Could you check a few things on this model? Use its own coordinates, in mm. Face numbers are marked on the shaded views. Round coordinates to 2 decimals unless told otherwise and drop trailing zeros. Loops run counter-clockwise (first coordinate to the right, second up) from the corner with the lowest first, then second, coordinate; pieces in that order, holes last. Notation, with made-up numbers: (10.25, 14) -> (68.25, 14) arc R18 cw to (68.25, 45) -> close; hole circle Ø1 at (2.25, 84.5). An arc over 180 degrees is marked (long way). Put each result on its own line as item: value. Start each with the question number.
1. I'm going to push flat-ended pins straight in: P1, Ø4, axis at y = -7, z = 5, coming from the -X side; P2, Ø4, axis at y = 7, z = 76.5, coming from the +X side; P3, Ø1, axis at x = -1, z = 60.5, coming from the +Y side. Where does each tip first touch, or does it pass through?
2. Imagine slicing it at B-B, the plane x = 0. Please give me the cut outline in (y, z), and give its area (3 significant figures).
3. I need wall thicknesses on line 1 (Z direction, x = 15.5, y = 4); line 2 (Y direction, x = 13, z = 103.6); line 3 (Y direction, x = -13, z = 101.8). Which ranges of each line are inside material? Lowest first, please. Write a range as [from, to].
4. Imagine slicing it at D-D, the plane x = 12.5. Please give me the cut outline in (y, z).
5. Imagine slicing it at A-A, the plane x = -13. Please give me the cut outline in (y, z), and give its area (3 significant figures).
6. If we mould it in two halves opening along Z, with no side actions, what happens to the marked faces 1, 2, 3 and 4? For each: pulls with the +Z half, pulls with the -Z half, needs draft (parallel to the pull), parting line crosses it, or undercut.
```python
from build123d import *

# Parameters (mm, degrees)
ESQUISSE1_R             = 10
BOSS_EXTRU_1_DEPTH      = 100
ESQUISSE2_R             = 17.5
BOSS_EXTRU_2_DEPTH      = 30
ESQUISSE3_W             = 40
ESQUISSE3_H             = 40
BOSS_EXTRU_3_DEPTH      = 5
ESQUISSE4_R             = 2.5
ENL_V_MAT_EXTRU_1_DEPTH = 5
ESQUISSE5_OUTSIDE_W     = 71.274
ESQUISSE5_OUTSIDE_H     = 71.274
ESQUISSE5_OUTSIDE_R     = 10
ENL_V_MAT_EXTRU_3_DEPTH = 20


with BuildPart() as part:
    # Esquisse1 → Boss.-Extru.1 (new body)
    with BuildSketch(Plane.XY):
        Circle(ESQUISSE1_R)
    extrude(amount=BOSS_EXTRU_1_DEPTH)

    # Esquisse2 → Boss.-Extru.2 (add)
    with BuildSketch(Plane(origin=(0, 0, 0), x_dir=(-1, 0, 0), z_dir=(0, 0, -1))):
        Circle(ESQUISSE2_R)
    extrude(amount=BOSS_EXTRU_2_DEPTH)

    # Esquisse3 → Boss.-Extru.3 (add)
    with BuildSketch(Plane.XY.offset(100)):
        Rectangle(ESQUISSE3_W, ESQUISSE3_H)
    extrude(amount=BOSS_EXTRU_3_DEPTH)

    # Esquisse4 → Enlèv. mat.-Extru.1 (cut)
    with BuildSketch(Plane.XY.offset(105)):
        with Locations((-13, 13)):
            Circle(ESQUISSE4_R)
        with Locations((13, -13)):
            Circle(ESQUISSE4_R)
    extrude(amount=-ENL_V_MAT_EXTRU_1_DEPTH, mode=Mode.SUBTRACT)

    # Esquisse5 outside → Enlèv. mat.-Extru.3 (cut)
    with BuildSketch(Plane.XY):
        Rectangle(ESQUISSE5_OUTSIDE_W, ESQUISSE5_OUTSIDE_H)
        Circle(ESQUISSE5_OUTSIDE_R, mode=Mode.SUBTRACT)
    extrude(amount=-ENL_V_MAT_EXTRU_3_DEPTH, mode=Mode.SUBTRACT)


solid = part.part
```
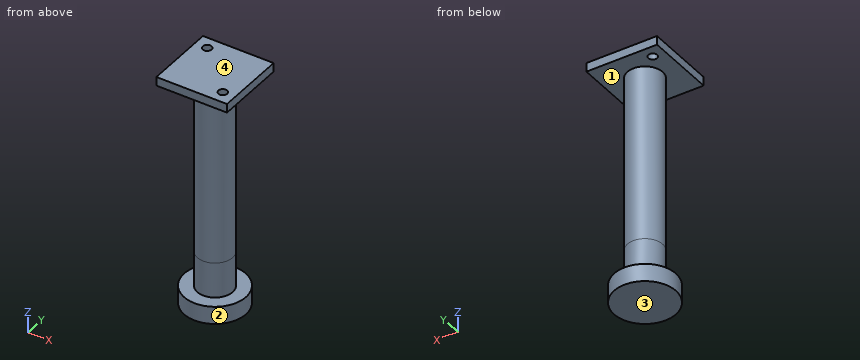
Entries:
1. P1: x = -8.66
1. P2: x = 8.66
1. P3: y = 9.99
2. outline: (-20, 100) -> (-10, 100) -> (-10, -20) -> (-17.5, -20) -> (-17.5, -30) -> (17.5, -30) -> (17.5, -20) -> (10, -20) -> (10, 100) -> (20, 100) -> (20, 105) -> (-20, 105) -> close
2. area: 2,950 mm^2
3. line 1: [-30, -20], [100, 105]
3. line 2: [-20, -15.5], [-10.5, 20]
3. line 3: [-20, 10.5], [15.5, 20]
4. outline: (-20, 100) -> (-15.45, 100) -> (-15.45, 105) -> (-20, 105) -> close; (-12.25, -30) -> (12.25, -30) -> (12.25, -20) -> (-12.25, -20) -> close; (-10.55, 100) -> (20, 100) -> (20, 105) -> (-10.55, 105) -> close
5. outline: (-20, 100) -> (10.5, 100) -> (10.5, 105) -> (-20, 105) -> close; (-11.72, -30) -> (11.72, -30) -> (11.72, -20) -> (-11.72, -20) -> close; (15.5, 100) -> (20, 100) -> (20, 105) -> (15.5, 105) -> close
5. area: 409 mm^2
6. face 1: undercut
6. face 2: needs draft
6. face 3: pulls with the -Z half
6. face 4: pulls with the +Z half
